from build123d import *

# Parameters (mm, degrees)
F1_DEPTH = 3.175


# Not quite as in the source:
# - a length typed as a fraction of an inch, garbled in the dataset ("3 / 203.2 mm" for 3/8 in), is restored


with BuildPart() as f1:
    # F0 (on Top) → F1 (new body)
    with BuildSketch(Plane.XY):
        Polygon((247.5, 123.5), (-247.5, 123.5), (-247.5, 0), (-190, 0), (-190, 60), (-160, 60), (-160, 0), (-102.5, 0), (-102.5, 60), (-72.5, 60), (-72.5, 0), (-15, 0), (-15, 60), (15, 60), (15, 0), (72.5, 0), (72.5, 60), (102.5, 60), (102.5, 0), (160, 0), (160, 60), (190, 60), (190, 0), (247.5, 0), align=None)
        Polygon((-190, 0), (-247.5, 0), (-247.5, -123.5), (247.5, -123.5), (247.5, 0), (190, 0), (190, -60), (160, -60), (160, 0), (102.5, 0), (102.5, -60), (72.5, -60), (72.5, 0), (15, 0), (15, -60), (-15, -60), (-15, 0), (-72.5, 0), (-72.5, -60), (-102.5, -60), (-102.5, 0), (-160, 0), (-160, -60), (-190, -60), align=None)
    extrude(amount=-F1_DEPTH)


solid = f1.part
Here's how the part is built. I have some questions about the finished solid (model axes, mm). Give positions to 0.01 mm unless a question says otherwise; leave off trailing zeros. Order: outer loops, then holes, each group sorted by start corner. A loop starts at its lowest first (then second) coordinate and runs counter-clockwise, first axis right, second up. Notation, with made-up numbers: (78, 64) -> (83, 64) arc R20 ccw to (83, 87) -> close; hole circle Ø5 at (-13.5, 68). An arc over 180 degrees is marked (long way). Use a Markdown table: item, result. Add a question column.
Item 1: Will this pin go through, and if not, where does the flat tip stop? pin 1 (12 mm diameter, centred on x = -49.5, y = 5.5, fed in from +Z).
Item 2: Imagine slicing it at A-A on x = 172.5. Please give me the cut outline in (y, z) (3 decimals).
Item 3: I need wall thicknesses on line 1 (X direction, y = 9, z = -1.8); line 2 (Y direction, x = -79.5, z = -1.95). Which ranges of each line are inside material? Lowest first, please.
Item 4: Imagine slicing it at B-B on y = -39.5. Please give me the cut outline in (x, z) (3 decimals).
Item 5: Imagine slicing it at C-C on z = -1.2. Please give me the cut outline in (x, y), plus the area to 3 significant figures.
Data:
| question | item | result |
|---|---|---|
| 1 | pin 1 | stops at z = 0 |
| 2 | outline | (-123.5, -3.175) -> (-60, -3.175) -> (-60, 0) -> (-123.5, 0) -> close; (60, -3.175) -> (123.5, -3.175) -> (123.5, 0) -> (60, 0) -> close |
| 3 | line 1 | x = -247.5 to -190, -160 to -102.5, -72.5 to -15, 15 to 72.5, 102.5 to 160, 190 to 247.5 |
| 3 | line 2 | y = -123.5 to -60, 60 to 123.5 |
| 4 | outline | (-247.5, -3.175) -> (-190, -3.175) -> (-190, 0) -> (-247.5, 0) -> close; (-160, -3.175) -> (-102.5, -3.175) -> (-102.5, 0) -> (-160, 0) -> close; (-72.5, -3.175) -> (-15, -3.175) -> (-15, 0) -> (-72.5, 0) -> close; (15, -3.175) -> (72.5, -3.175) -> (72.5, 0) -> (15, 0) -> close; (102.5, -3.175) -> (160, -3.175) -> (160, 0) -> (102.5, 0) -> close; (190, -3.175) -> (247.5, -3.175) -> (247.5, 0) -> (190, 0) -> close |
| 5 | outline | (-247.5, -123.5) -> (247.5, -123.5) -> (247.5, 123.5) -> (-247.5, 123.5) -> close; hole (-190, -60) -> (-160, -60) -> (-160, 60) -> (-190, 60) -> close; hole (-102.5, -60) -> (-72.5, -60) -> (-72.5, 60) -> (-102.5, 60) -> close; hole (-15, -60) -> (15, -60) -> (15, 60) -> (-15, 60) -> close; hole (72.5, -60) -> (102.5, -60) -> (102.5, 60) -> (72.5, 60) -> close; hole (160, -60) -> (190, -60) -> (190, 60) -> (160, 60) -> close |
| 5 | area | 104,000 mm² |
